```python
from build123d import *

# Parameters (mm, degrees)
SKETCH1_R           = 1.5
BOSS_EXTRUDE1_DEPTH = 20
CUT_EXTRUDE1_DEPTH  = 2
CUT_EXTRUDE2_START  = 20
CUT_EXTRUDE2_DEPTH  = 2


with BuildPart() as part:
    # Sketch1 → Boss-Extrude1 (new body)
    with BuildSketch(Plane(origin=(0, 0, 0), x_dir=(0, 0, -1), z_dir=(1, 0, 0))):
        with BuildLine():
            Line((-24.25, -4), (3, -4))
            ThreePointArc((3, -4), (4.414213562, -3.414213562), (5, -2))
            Line((5, -2), (5, 15.754424432))
            ThreePointArc((5, 15.754424432), (4.439006977, 17.143402085), (3.070741081, 17.753172966))
            ThreePointArc((3.070741081, 17.753172966), (-14.52537265, 12.863616062), (-26.106953382, -1.257218647))
            ThreePointArc((-26.106953382, -1.257218647), (-25.906134461, -3.121257619), (-24.25, -4))
        make_face()
        with Locations((0, 7.792107243)):
            Circle(SKETCH1_R, mode=Mode.SUBTRACT)
        Circle(SKETCH1_R, mode=Mode.SUBTRACT)
        with Locations((-11.694197133, 0)):
            Circle(SKETCH1_R, mode=Mode.SUBTRACT)
        with BuildLine():
            Line((-16.194197133, 0), (-19.086908103, 0))
            ThreePointArc((-19.086908103, 0), (-19.523483355, 0.256274644), (-19.512525938, 0.762391804))
            ThreePointArc((-19.512525938, 0.762391804), (-18.131084667, 2.778063971), (-16.561428533, 4.650894419))
            ThreePointArc((-16.561428533, 4.650894419), (-16.012010004, 4.777196244), (-15.694197133, 4.311569945))
            Line((-15.694197133, 4.311569945), (-15.694197133, 0.5))
            ThreePointArc((-15.694197133, 0.5), (-15.840643743, 0.146446609), (-16.194197133, 0))
        make_face(mode=Mode.SUBTRACT)
        with BuildLine():
            Line((-11.408525011, 8.313239357), (-6.562071453, 1.068743928))
            ThreePointArc((-6.562071453, 1.068743928), (-6.037987222, 0.85867559), (-5.652264441, 1.2709994))
            Line((-5.652264441, 1.2709994), (-4.115149007, 11.298363901))
            ThreePointArc((-4.115149007, 11.298363901), (-4.277279765, 11.747905828), (-4.742779484, 11.855999947))
            ThreePointArc((-4.742779484, 11.855999947), (-8.099246212, 10.666463574), (-11.255194335, 9.016961489))
            ThreePointArc((-11.255194335, 9.016961489), (-11.481482966, 8.697701132), (-11.408525011, 8.313239357))
        make_face(mode=Mode.SUBTRACT)
    extrude(amount=BOSS_EXTRUDE1_DEPTH)

    # Sketch2 → Cut-Extrude1 (cut)
    with BuildSketch(Plane(origin=(0, 0, 0), x_dir=(0, 0, -1), z_dir=(1, 0, 0))):
        Polygon((-11.694197133, -3.233161507), (-8.894197133, -1.616580754), (-8.894197133, 1.616580754), (-11.694197133, 3.233161507), (-14.494197133, 1.616580754), (-14.494197133, -1.616580754), align=None)
        Polygon((0, -3.233161507), (2.8, -1.616580754), (2.8, 1.616580754), (0, 3.233161507), (-2.8, 1.616580754), (-2.8, -1.616580754), align=None)
        Polygon((0, 4.558945735), (2.8, 6.175526489), (2.8, 9.408687997), (0, 11.02526875), (-2.8, 9.408687997), (-2.8, 6.175526489), align=None)
    extrude(amount=CUT_EXTRUDE1_DEPTH, mode=Mode.SUBTRACT)

    # Sketch2<2> → Cut-Extrude2 (cut)
    with BuildSketch(Plane(origin=(0, 0, 0), x_dir=(0, 0, -1), z_dir=(1, 0, 0)).offset(CUT_EXTRUDE2_START)):
        Polygon((-11.694197133, -3.233161507), (-8.894197133, -1.616580754), (-8.894197133, 1.616580754), (-11.694197133, 3.233161507), (-14.494197133, 1.616580754), (-14.494197133, -1.616580754), align=None)
        Polygon((0, -3.233161507), (2.8, -1.616580754), (2.8, 1.616580754), (0, 3.233161507), (-2.8, 1.616580754), (-2.8, -1.616580754), align=None)
        Polygon((0, 4.558945735), (2.8, 6.175526489), (2.8, 9.408687997), (0, 11.02526875), (-2.8, 9.408687997), (-2.8, 6.175526489), align=None)
    extrude(amount=-CUT_EXTRUDE2_DEPTH, mode=Mode.SUBTRACT)


solid = part.part
```
Geometry: final body of the model. Coordinates: model frame, mm. A direction names the side the tool comes from. Round coordinates to 2 decimals unless told otherwise and drop trailing zeros. Write each loop counter-clockwise with the first axis right and the second up, starting at its lowest first coordinate (ties: lowest second). Pieces come first, ordered by that corner, then holes. Notation, with made-up numbers: M -3,-28.5 L 2,-28.5 A24 ccw 2,8.5 Z; hole C 12.5,30.5 d9. An arc over 180 degrees is marked long. Answer in a Markdown table with one row per item. Add a question column.
(1) Cut plane D-D, the plane z = 9.5. Return the cut outline in (x, y).
(2) Ray query, L1, parallel to Z at x = 14.25, y = 7.5; L2, parallel to Z at x = 11, y = 4.5; L3, parallel to Y at x = 8.5, z = 0. Return the intervals inside material, ascending.
(3) Cut plane A-A, the plane y = -0.5. Return the cut outline in (x, z), then the cut area to 3 significant figures.
(4) Draft query along Y for faces 1 (the face through (19.01, 2.41, 10.27)), 2 (the face through (0, 7, 11)), 3 (the face through (10, -4, 11)), 4 (the face through (9.86, 4.74, 9.02)). Return one class per face: pulls with the +Y half, pulls with the -Y half, needs draft (parallel to the pull), parting line crosses it, or undercut.
(5) Cut plane C-C, the plane z = -1. Return the cut outline in (x, y).
(6) Reachability of faces 5 (the face through (9.86, 2.75, 18.15)), 6 (the face through (19, 0, 2.8)), 7 (the face through (1, 0, 8.894)) from +Z, -Z, +X, -X, +Y, -Y: full face, straight path, thin tool, end or side. Return the list, or none.
(7) Cut plane B-B, the plane x = 13.5. Return the cut outline in (y, z).
(8) Contact query for flat-ended pins moving along their axis: pin 1 (3.5 mm diameter, centred on y = 7.79, z = 0, fed in from +X); pin 2 (2 mm diameter, centred on x = 19, y = 0.5, fed in from +Z); pin 3 (3 mm diameter, centred on x = 14.5, y = 14.5, fed in from +Z). Output: stop coordinate, or through.
Established:
| question | item | result |
|---|---|---|
| 1 | outline | M 0,-4 L 20,-4 L 20,-1.97 L 18,-1.97 L 18,1.97 L 20,1.97 L 20,5.46 L 0,5.46 L 0,1.97 L 2,1.97 L 2,-1.97 L 0,-1.97 Z; M 0,10 L 20,10 L 20,15.5 L 0,15.5 Z |
| 2 | L1 | -5 to -1.47, 1.47 to 4.7, 10.86 to 20.72 |
| 2 | L2 | -5 to 5.16, 8.86 to 15.73, 16.7 to 23.05 |
| 2 | L3 | -4 to -1.5, 1.5 to 6.29, 9.29 to 17.71 |
| 3 | outline | M 0,-5 L 20,-5 L 20,-2.8 L 18,-2.8 L 18,-1.41 L 2,-1.41 L 2,-2.8 L 0,-2.8 Z; M 0,2.8 L 2,2.8 L 2,1.41 L 18,1.41 L 18,2.8 L 20,2.8 L 20,8.89 L 18,8.89 L 18,10.28 L 2,10.28 L 2,8.89 L 0,8.89 Z; M 0,14.49 L 2,14.49 L 2,13.11 L 18,13.11 L 18,14.49 L 20,14.49 L 20,25.79 L 0,25.79 Z |
| 3 | area | 481 mm² |
| 4 | face 1 | undercut |
| 4 | face 2 | needs draft |
| 4 | face 3 | pulls with the -Y half |
| 4 | face 4 | undercut |
| 5 | outline | M 0,-4 L 20,-4 L 20,-2.66 L 18,-2.66 L 18,-1.12 L 2,-1.12 L 2,-2.66 L 0,-2.66 Z; M 0,2.66 L 2,2.66 L 2,1.12 L 18,1.12 L 18,2.66 L 20,2.66 L 20,5.14 L 18,5.14 L 18,6.67 L 2,6.67 L 2,5.14 L 0,5.14 Z; M 0,10.45 L 2,10.45 L 2,8.91 L 18,8.91 L 18,10.45 L 20,10.45 L 20,17.76 L 0,17.76 Z |
| 6 | face 5 | +X, -X |
| 6 | face 6 | +X |
| 6 | face 7 | -X |
| 7 | outline | M -4,-3 A2 ccw -2,-5 L 15.75,-5 A2 ccw 17.75,-3.07 A30.27 ccw -1.26,26.11 A2 ccw -4,24.25 Z; hole C 0,0 d3; hole C 0,11.69 d3; hole M 0,16.19 A0.5 ccw 0.5,15.69 L 4.31,15.69 A0.5 ccw 4.65,16.56 A25.27 ccw 0.76,19.51 A0.5 ccw 0,19.09 Z; hole M 1.07,6.56 A0.5 ccw 1.27,5.65 L 11.3,4.12 A0.5 ccw 11.86,4.74 A25.27 ccw 9.02,11.26 A0.5 ccw 8.31,11.41 Z; hole C 7.79,0 d3 |
| 8 | pin 1 | x = 18 |
| 8 | pin 2 | z = 25.79 |
| 8 | pin 3 | z = 14.31 |
